from build123d import *

# Parameters (mm, degrees)
F0_R     = 5.085
F1_DEPTH = 7.24
F2_R     = 5
F3_R     = 3.87
F4_DEPTH = 4
F5_SIZE  = 0.5


with BuildPart() as f1:
    # F0 (on Top) → F1 (new body)
    with BuildSketch(Plane.XY):
        Circle(F0_R)
    extrude(amount=F1_DEPTH)

    # F2
    f2_edges = [f1.edges().sort_by_distance(p)[0] for p in [
        (-5.085, 0, 7.24),
    ]]
    fillet(f2_edges, radius=F2_R)

    # F3 (on face) → F4 (join)
    with BuildSketch(Plane(origin=(0, 0, 0), x_dir=(1, 0, 0), z_dir=(0, 0, -1))):
        Circle(F3_R)
    extrude(amount=F4_DEPTH)

    # F5
    f5_edges = [f1.edges().sort_by_distance(p)[0] for p in [
        (-3.87, 0, -4),
    ]]
    chamfer(f5_edges, length=F5_SIZE)


solid = f1.part
Could you check a few things on this model? Use its own coordinates, in mm. A direction names the side the tool comes from. Give positions to 0.01 mm unless a question says otherwise; leave off trailing zeros. Order: outer loops, then holes, each group sorted by start corner. A loop starts at its lowest first (then second) coordinate and runs counter-clockwise, first axis right, second up.
1. Which directions (+Z, -Z, +X, -X, +Y, -Y) give clear straight access to the entire face, cutting with the end or side of a thin tool? Please do faces 1 (the cylindrical face through (2.73, 4.29, 1.1)), 2 (the flat face through (-1, -4, 0)).
Answers below:
face 1: +Z, -Z
face 2: -Z
2. Suppose I cut it at A-A (z = -1.5). Write out the boundary of the cut face in (x, y).
Answers below:
outline: circle Ø7.74 at (0, 0)
3. For pin 1 (4 mm diameter, centred on x = 0.5, y = 4, fed in from +Z); pin 2 (5 mm diameter, centred on y = 3.5, z = -3, fed in from -X), each with a flat end and sliding along its axis, tell me the tip position at first contact or that it passes through.
Answers below:
pin 1: stops at z = 6.85
pin 2: stops at x = -3.74
4. I need wall thicknesses on L1, parallel to Z at x = 1, y = 1.25; L2, parallel to Z at x = -4.5, y = -1.5; L3, parallel to X at y = -0.5, z = 6.5. Which ranges of each line are inside material? Lowest first, please.
Answers below:
L1: z = -4 to 7
L2: z = 0 to 4.06
L3: x = -2.66 to 2.66
